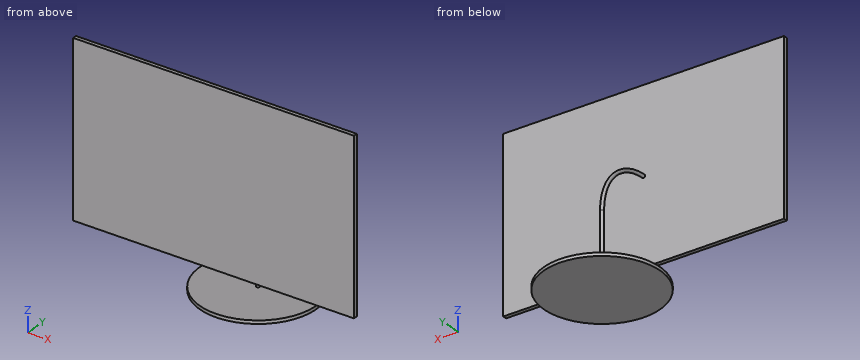
from build123d import *

# Parameters (mm, degrees)
F0_W     = 541.02
F0_H     = 325.12
F1_DEPTH = 7.62
F3_R     = 3.175
F5_R     = 110.49
F5_R_2   = 3.175
F6_DEPTH = 6.35


with BuildPart() as f1:
    # F0 (on Front) → F1 (new body)
    with BuildSketch(Plane.XZ):
        Rectangle(F0_W, F0_H)
    extrude(amount=F1_DEPTH)

    # F4: sweep along a path in F2
    with BuildLine(Plane.YZ) as f4_path:
        ThreePointArc((0, 0), (78.1282282533, -32.3617717467), (110.49, -110.49))
        Line((110.49, -110.49), (110.49, -251.46))
    # F3 (on face) → F4 (sweep)
    with BuildSketch(Plane(origin=(0, 0, 0), x_dir=(-1, 0, 0), z_dir=(0, 1, 0))):
        Circle(F3_R)
    sweep(path=f4_path.line)

    # F5 (on face) → F6 (join)
    with BuildSketch(Plane(origin=(0, 0, -251.46), x_dir=(1, 0, 0), z_dir=(0, 0, -1))):
        with Locations((0, -110.49)):
            Circle(F5_R)
        with Locations((0, -110.49)):
            Circle(F5_R_2, mode=Mode.SUBTRACT)
    extrude(amount=-F6_DEPTH)


solid = f1.part
Geometry: final body of the model. Coordinates: model frame, mm. Coordinates: 2 decimals unless noted, no trailing zeros. Loops run counter-clockwise (first coordinate to the right, second up) from the corner with the lowest first, then second, coordinate; pieces in that order, holes last. Notation, with made-up numbers: M -16.75,-33.75 L -12.75,-33.75 A15 ccw -12.75,-15.75 Z; hole C -33.75,15.25 d2. An arc over 180 degrees is marked long. One line per item, written item: value. Start each with the question number.
1) Material intervals for L1, parallel to Y at x = -107, z = -121.5; L2, parallel to Z at x = 53, y = 51.5; L3, parallel to X at y = 84.5, z = -37, sorted ascending. Write a range as from..to.
2) Pin query (flat end, axial travel): P1, Ø8.5, axis at x = -103.5, y = -5.5, coming from the -Z side; P2, Ø10, axis at x = -30, y = 132.5, coming from the +Z side. Return the tip coordinate at first contact, or that it passes through.
3) Cut plane A-A (x = -18). Return loops of the section in (y, z).
4) Cut plane C-C (x = -153). Return loops of the section in (y, z).
5) Cut plane D-D (x = -91.5). Return loops of the section in (y, z), then the cut area to 3 significant figures.
6) Cut plane B-B (z = 126.5). Return loops of the section in (x, y).
Evaluation:
1. L1: -7.62..0
1. L2: -251.46..-245.11
1. L3: -2.8..2.8
2. P1: z = -162.56
2. P2: z = -245.11
3. outline: M -7.62,-162.56 L 0,-162.56 L 0,162.56 L -7.62,162.56 Z; M 1.48,-251.46 L 219.5,-251.46 L 219.5,-245.11 L 1.48,-245.11 Z
4. outline: M -7.62,-162.56 L 0,-162.56 L 0,162.56 L -7.62,162.56 Z
5. outline: M -7.62,-162.56 L 0,-162.56 L 0,162.56 L -7.62,162.56 Z; M 48.56,-251.46 L 172.42,-251.46 L 172.42,-245.11 L 48.56,-245.11 Z
5. area: 3,260 mm^2
6. outline: M -270.51,-7.62 L 270.51,-7.62 L 270.51,0 L -270.51,0 Z
